Can you work these out from the model? Positions are in its coordinate system, mm. A direction names the side the tool comes from. Round coordinates to 2 decimals unless told otherwise and drop trailing zeros. Order: outer loops, then holes, each group sorted by start corner. A loop starts at its lowest first (then second) coordinate and runs counter-clockwise, first axis right, second up. Notation, with made-up numbers: (2.25, 5) -> (57.25, 5) arc R13 cw to (57.25, 24) -> close; hole circle Ø6 at (29, 60.5). An arc over 180 degrees is marked (long way). Use a Markdown table: item, result. Add a question column.
Q1. If we section it at B-B on z = 0: List the corners of the cut face in (x, y) for me, plus the area to 3 significant figures.
Q2. I'm going to push flat-ended pins straight in: pin 1 Ø6 at (x, z) = (75.5, 200.5) entering from -Y; pin 2 Ø10 at (x, y) = (20, -227) entering from -Z; pin 3 Ø2 at (x, y) = (98.5, 156.5) entering from -Z. Where does each tip first touch, or does it pass through?
Q3. For faces 1 (the face through (199.65, -23.846, -107.384)), 2 (the face through (119, -2, 135)), 3 (the face through (119, 135, -2)), 4 (the face through (-175, -2, 2)), 5 (the face through (-23.846, -218.655, -107.384)), which set-ups out of +Z, -Z, +X, -X, +Y, -Y let a thin tool reach every point of the face, with its end or its side?
Q4. If we section it at D-D on z = 123.5: List the corners of the cut face in (x, y) for me, plus the area to 3 significant figures.
Q5. I need wall thicknesses on line 1 along X through (y, z) = (-120, 43); line 2 along Z through (x, y) = (169, -31). Which ranges of each line are inside material? Lowest first, please. Write a range as [from, to].
Q6. If we section it at C-C on y = 0: List the corners of the cut face in (x, z) for me.
Q7. If we section it at A-A on x = 0: List the corners of the cut face in (y, z) for me, plus the area to 3 significant figures.
```python
from build123d import *

# Parameters (mm, degrees)
F0_R     = 110
F1_DEPTH = 300
F2_R     = 110
F3_DEPTH = 300
F4_W     = 270
F4_H     = 270
F5_DEPTH = 175
F6_R     = 110
F7_DEPTH = 50


with BuildPart() as f1:
    # F0 (on Front) → F1 (new body, symmetric)
    with BuildSketch(Plane.XZ):
        Circle(F0_R)
    extrude(amount=F1_DEPTH, both=True)

    # F2 (on Top) → F3 (join)
    with BuildSketch(Plane.XY):
        Circle(F2_R)
    extrude(amount=F3_DEPTH)

    # F4 (on Right) → F5 (join, symmetric)
    with BuildSketch(Plane.YZ):
        Rectangle(F4_W, F4_H)
    extrude(amount=F5_DEPTH, both=True)

    # F6 (on face) → F7 (join)
    with BuildSketch(Plane.YZ.offset(175)):
        Circle(F6_R)
    extrude(amount=F7_DEPTH)


solid = f1.part
```
Answer below:
| question | item | result |
|---|---|---|
| 1 | outline | (-175, -135) -> (-110, -135) -> (-110, -300) -> (110, -300) -> (110, -135) -> (175, -135) -> (175, -110) -> (225, -110) -> (225, 110) -> (175, 110) -> (175, 135) -> (110, 135) -> (110, 300) -> (-110, 300) -> (-110, 135) -> (-175, 135) -> close |
| 1 | area | 178,000 mm² |
| 2 | pin 1 | y = -82.73 |
| 2 | pin 2 | z = -108.97 |
| 2 | pin 3 | z = -50.93 |
| 3 | face 1 | +X |
| 3 | face 2 | +Z |
| 3 | face 3 | +Y |
| 3 | face 4 | +Z, -Z, -X, +Y, -Y |
| 3 | face 5 | -Y |
| 4 | outline | (-175, -135) -> (175, -135) -> (175, 135) -> (-175, 135) -> close |
| 4 | area | 94,500 mm² |
| 5 | line 1 | [-175, 175] |
| 5 | line 2 | [-135, 135] |
| 6 | outline | (-175, -135) -> (175, -135) -> (175, -110) -> (225, -110) -> (225, 110) -> (175, 110) -> (175, 135) -> (110, 135) -> (110, 300) -> (-110, 300) -> (-110, 135) -> (-175, 135) -> close |
| 7 | outline | (-300, -110) -> (-135, -110) -> (-135, -135) -> (135, -135) -> (135, -110) -> (300, -110) -> (300, 110) -> (135, 110) -> (135, 135) -> (110, 135) -> (110, 300) -> (-110, 300) -> (-110, 135) -> (-135, 135) -> (-135, 110) -> (-300, 110) -> close |
| 7 | area | 182,000 mm² |
